CAD build for the part. Positions are in the model's coordinates, mm. A direction names the side the tool comes from. Round coordinates to 2 decimals unless told otherwise and drop trailing zeros. Order: outer loops, then holes, each group sorted by start corner. A loop starts at its lowest first (then second) coordinate and runs counter-clockwise, first axis right, second up. Notation, with made-up numbers: (85.25, -32) -> (137.25, -32) arc R22 ccw to (137.25, -20) -> close; hole circle Ø2 at (9.25, 77.5). An arc over 180 degrees is marked (long way). Return JSON: item names as keys, results as strings. Group by question number.
Q1. Cut at B-B (z = -7.5). Write the cut outline in (x, y), then the cut area to 3 significant figures.
Q2. Which spindle directions (+Z, -Z, +X, -X, +Y, -Y) get a long thin tool onto all of the face, cutting with end or side? Do faces 1 (the cylindrical face through (8.85, 21.23, -6.36)), 2 (the flat face through (0, 17, -5)), 3 (the flat face through (-2, 14, -5)), 4 (the flat face through (23, 14, -5)), 5 (the flat face through (23, 15, -5)). Say none if no direction does.
Q3. Cut at A-A (y = 16.5). Write the cut outline in (x, z).
Q4. Probe line 1 along Z through (x, y) = (4.6, 11); line 2 along X through (y, z) = (8.5, -4.6); line 3 along Y through (x, z) = (19.75, -6). List the from-to ranges inside material, lowest first.
Q5. Flat gauge pins, fed straight in: pin 1 (4 mm diameter, centred on y = 9.5, z = -3.5, fed in from -X); pin 2 (1.8 mm diameter, centred on x = 22.5, z = -6.5, fed in from +Y); pin 3 (4.5 mm diameter, centred on y = 6.5, z = -3.5, fed in from +X). Where does each tip first touch, or does it go through?
Q6. Cut at C-C (z = -5.5). Write the cut outline in (x, y), then the cut area to 3 significant figures.
Q7. Cut at D-D (x = 2.25). Write the cut outline in (y, z).
Autodesk Inventor part; units mm, degrees
ref_plane "YZ Plane" through (0, 0, 0) normal (1, 0, 0) x (0, 1, 0)
ref_plane "XZ Plane" through (0, 0, 0) normal (0, 1, 0) x (-1, 0, 0)
ref_plane "XY Plane" through (0, 0, 0) normal (0, 0, 1) x (1, 0, 0)
sketch "スケッチ1" plane through (0, 0, 0) normal (0, 1, 0) x (-1, 0, 0)
  line L0 (0, 0) -> (-21, 0)
  line L1 (-21, 0) -> (-21, -9.2)
  line L2 (-21, -9.2) -> (0, -9.2)
  line L3 (0, -9.2) -> (0, 0)
  dimension "d0" = 21
  dimension "d1" = 9.2
extrude "押し出し1" add sketch "スケッチ1" along normal blind 14
sketch "スケッチ2" plane through (0, 14, 0) normal (0, 1, 0) x (1, 0, 0)
  line L0 (21, 0) -> (21, 9.2)
  line L1 (21, 9.2) -> (0, 9.2)
  line L2 (0, 9.2) -> (0, 0)
  line L3 (0, 0) -> (21, 0)
  line L4 (-3.5, 0) -> (24.5, 0)
  line L5 (24.5, 0) -> (24.5, 9.2)
  line L6 (24.5, 9.2) -> (-3.5, 9.2)
  line L7 (-3.5, 9.2) -> (-3.5, 0)
  dimension "d4" = 3.5
  dimension "d5" = 3.5
extrude "押し出し2" add sketch "スケッチ2" along normal blind 1
sketch "スケッチ3" plane through (0, 15, 0) normal (0, 1, 0) x (1, 0, 0)
  line L0 (-3.5, 0) -> (24.5, 0)
  line L1 (24.5, 9.2) -> (-3.5, 9.2)
  line L2 (0, 9.2) -> (0, 0)
  line L3 (21, 0) -> (21, 9.2)
extrude "押し出し3" add sketch "スケッチ3" along normal blind 4.5
sketch "スケッチ4" plane through (0, 19.5, 0) normal (0, 1, 0) x (1, 0, 0)
  line L0 (21, 9.2) -> (0, 9.2)
  line L1 (0, 9.2) -> (0, 0)
  line L2 (0, 0) -> (21, 0)
  circle A0 centre (4.6, 4.6) radius 4.6
extrude "押し出し4" add sketch "スケッチ4" along normal blind 3.5 contours A0
sketch "スケッチ5" plane through (4.6, 23, -4.6) normal (0, 1, 0) x (1, 0, 0)
  circle A0 centre (0, 0) radius 4.6
  point P0 (-4.6, -4.6)
hole "穴1" at (4.6, 23, -4.6) direction (0, -1, 0) diameter 3 end through all
equation "\"d5\" = d4"
properties part number "motor"
Solution:
{
 "1": {"outline": "(-3.5, 14) -> (0, 14) -> (0, 0) -> (21, 0) -> (21, 14) -> (24.5, 14) -> (24.5, 15) -> (21, 15) -> (21, 19.5) -> (8.17, 19.5) -> (8.17, 23) -> (1.03, 23) -> (1.03, 19.5) -> (0, 19.5) -> (0, 15) -> (-3.5, 15) -> close", "area": "441 mm²"},
 "2": {"face 1": "+Y", "face 2": "+Z, -Z, -X, +Y", "face 3": "+Z, -Z, -X, -Y", "face 4": "+Z, -Z, +X, -Y", "face 5": "+Z, -Z, +X, +Y"},
 "3": {"outline": "(0, -9.2) -> (21, -9.2) -> (21, 0) -> (0, 0) -> close; hole circle Ø3 at (4.6, -4.6)"},
 "4": {"line 1": "z = -9.2 to -6.1, -3.1 to 0", "line 2": "x = 0 to 3.1, 6.1 to 21", "line 3": "y = 0 to 19.5"},
 "5": {"pin 1": "stops at x = 0", "pin 2": "stops at y = 15", "pin 3": "stops at x = 21"},
 "6": {"outline": "(-3.5, 14) -> (0, 14) -> (0, 0) -> (3.4, 0) -> (3.4, 23) -> (0.09, 23) -> (0.09, 19.5) -> (0, 19.5) -> (0, 15) -> (-3.5, 15) -> close; (5.8, 0) -> (21, 0) -> (21, 14) -> (24.5, 14) -> (24.5, 15) -> (21, 15) -> (21, 19.5) -> (9.11, 19.5) -> (9.11, 23) -> (5.8, 23) -> close", "area": "393 mm²"},
 "7": {"outline": "(0, -9.2) -> (19.5, -9.2) -> (19.5, -8.55) -> (23, -8.55) -> (23, -0.65) -> (19.5, -0.65) -> (19.5, 0) -> (0, 0) -> close"}
}
